```python
from build123d import *

# Parameters (mm, degrees)
F1_DEPTH  = 7.8
F2_R      = 2.4
F3_DEPTH  = 1.7
F4_W      = 5.02
F4_H      = 4.92
F5_DEPTH  = 1.5
F6_W      = 4.16
F6_H      = 4.92
F7_DEPTH  = 7.9
F8_R      = 2.4
F8_R_2    = 2
F9_DEPTH  = 1.6
F10_DEPTH = 1
F11_W     = 5
F11_H     = 5.1
F12_DEPTH = 2


with BuildPart() as f1:
    # F0 (on Front) → F1 (new body)
    with BuildSketch(Plane.XZ):
        Polygon((0, 1.44), (0, 0), (7.9, 0), (7.9, 9.5), (1.5, 9.5), (1.5, 1.44), align=None)
    extrude(amount=F1_DEPTH)

    # F2 (on face) → F3 (join)
    with BuildSketch(Plane.XY.offset(9.5)):
        with Locations((4, -3.9)):
            Circle(F2_R)
    extrude(amount=F3_DEPTH)

    # F4 (on face) → F5 (cut)
    with BuildSketch(Plane(origin=(0, 0, 0), x_dir=(1, 0, 0), z_dir=(0, 0, -1))):
        with Locations((3.95, 3.9)):
            Rectangle(F4_W, F4_H)
    extrude(amount=-F5_DEPTH, mode=Mode.SUBTRACT)

    # F6 (on face) → F7 (cut)
    with BuildSketch(Plane(origin=(0, 0, 1.5), x_dir=(1, 0, 0), z_dir=(0, 0, -1))):
        with Locations((4.38, 3.9)):
            Rectangle(F6_W, F6_H)
    extrude(amount=-F7_DEPTH, mode=Mode.SUBTRACT)

    # F8 (on face) → F9 (join)
    with BuildSketch(Plane(origin=(1.5, 0, 0), x_dir=(0, -1, 0), z_dir=(-1, 0, 0))):
        with Locations((3.9, 5.47)):
            Circle(F8_R)
        with Locations((3.9, 5.47)):
            Circle(F8_R_2, mode=Mode.SUBTRACT)
    extrude(amount=F9_DEPTH)

    # F8 (on face) → F10 (cut)
    with BuildSketch(Plane(origin=(1.5, 0, 0), x_dir=(0, -1, 0), z_dir=(-1, 0, 0))):
        with Locations((3.9, 5.47)):
            Circle(F8_R_2)
    extrude(amount=-F10_DEPTH, mode=Mode.SUBTRACT)

    # F11 (on face) → F12 (cut)
    with BuildSketch(Plane.YZ.offset(7.9)):
        with Locations((-3.9, 5.55)):
            Rectangle(F11_W, F11_H)
    extrude(amount=-F12_DEPTH, mode=Mode.SUBTRACT)


solid = f1.part
```
The model under review builds one solid part; all positions refer to its coordinate system, in mm. A direction names the side the tool comes from. Round coordinates to 2 decimals unless told otherwise and drop trailing zeros. Write each loop counter-clockwise with the first axis right and the second up, starting at its lowest first coordinate (ties: lowest second). Pieces come first, ordered by that corner, then holes. Notation, with made-up numbers: (56.25, 75) - (73.25, 75) arc R21 cw to (73.25, 114) - close; hole circle Ø7 at (57, 6). An arc over 180 degrees is marked (long way). Answer as CSV lines item,"result". Start each with the question number.
(1) We need section A-A on z = 5.47. State the section outline as (x, y) points.
(2) We need section B-B on x = 0.5. State the section outline as (y, z) points, plus the area to 3 significant figures.
(3) Draft analysis for pull direction Z (two halves, no side actions). For faces 1 (the flat face through (4, -1.44, 5)), 2 (the flat face through (7, -6.4, 6)), 3 (the flat face through (4, -4, 11.2)), state which applies: pulls with the +Z half, pulls with the -Z half, needs draft (parallel to the pull), parting line crosses it, or undercut.
(4) We need section C-C on y = -3.9. State the section outline as (x, z) points.
(5) We need section D-D on x = 7. State the section outline as (y, z) points, plus the area to 3 significant figures.
(6) To check wall thickness, follow line 1 (Z direction, x = 0.35, y = -3.9); line 2 (X direction, y = -5.75, z = 2); line 3 (Z direction, x = 7.25, y = -1.5). State the ranges of each line that lie inside material, in increasing order.
(7) For pin 1 Ø1 at (x, y) = (7, -2.5) entering from +Z; pin 2 Ø1.6 at (y, z) = (-3.5, 1) entering from -X; pin 3 Ø1.4 at (y, z) = (-3, 9) entering from -X, all flat-tipped, find the tip position at first contact; note any pin that passes through.
(8) For faces 4 (the cylindrical face through (0.71, -5.01, 3.34)), 5 (the flat face through (6.46, -4, 9)), 6 (the flat face through (7, -1.4, 6)), 7 (the cylindrical face through (6.217, -4.819, 10.338)), 8 (the flat face through (1, -4, 1.44)), list the 3-axis set-ups (+Z, -Z, +X, -X, +Y, -Y) from which the entire face can be reached by the end or side of a thin tool; tool diameter is ignored.
Worked answers:
1,outline,"(-0.1, -6.3) - (1.5, -6.3) - (1.5, -7.8) - (7.9, -7.8) - (7.9, -6.4) - (5.9, -6.4) - (5.9, -6.36) - (2.3, -6.36) - (2.3, -5.9) - (-0.1, -5.9) - close; (-0.1, -1.9) - (2.3, -1.9) - (2.3, -1.44) - (5.9, -1.44) - (5.9, -1.4) - (7.9, -1.4) - (7.9, 0) - (1.5, 0) - (1.5, -1.5) - (-0.1, -1.5) - close"
2,outline,"(-7.8, 0) - (0, 0) - (0, 1.44) - (-7.8, 1.44) - close; circle Ø4.8 at (-3.9, 5.47); hole circle Ø4 at (-3.9, 5.47)"
2,area,"16.8 mm²"
3,face 1,"needs draft"
3,face 2,"undercut"
3,face 3,"pulls with the +Z half"
4,outline,"(-0.1, 3.07) - (1.5, 3.07) - (1.5, 1.5) - (2.3, 1.5) - (2.3, 3.47) - (-0.1, 3.47) - close; (-0.1, 7.47) - (2.3, 7.47) - (2.3, 9.4) - (6.46, 9.4) - (6.46, 8.1) - (7.9, 8.1) - (7.9, 9.5) - (6.4, 9.5) - (6.4, 11.2) - (1.6, 11.2) - (1.6, 9.5) - (1.5, 9.5) - (1.5, 7.87) - (-0.1, 7.87) - close; (0, 0) - (1.44, 0) - (1.44, 1.44) - (0, 1.44) - close; (6.46, 0) - (7.9, 0) - (7.9, 3) - (6.46, 3) - close"
5,outline,"(-7.8, 0) - (0, 0) - (0, 9.5) - (-7.8, 9.5) - close; hole (-6.4, 3) - (-1.4, 3) - (-1.4, 8.1) - (-6.4, 8.1) - close"
5,area,"48.6 mm²"
6,line 1,"0 to 1.44, 3.07 to 3.47, 7.47 to 7.87"
6,line 2,"1.5 to 2.3, 6.46 to 7.9"
6,line 3,"0 to 3, 8.1 to 9.5"
7,pin 1,"z = 9.5"
7,pin 2,"x = 0"
7,pin 3,"x = 1.5"
8,face 4,"-X"
8,face 5,"-Z"
8,face 6,"+X"
8,face 7,"+Z"
8,face 8,"-X, +Y, -Y"
